Build history of the part. All positions in model axes, mm. Coordinates: 2 decimals unless noted, no trailing zeros. Order: outer loops, then holes, each group sorted by start corner. A loop starts at its lowest first (then second) coordinate and runs counter-clockwise, first axis right, second up. Notation, with made-up numbers: (35, 65.5) - (49, 65.5) arc R17 cw to (49, 74.5) - close; hole circle Ø8 at (43, 14.5). An arc over 180 degrees is marked (long way). One line per item, written item: value.
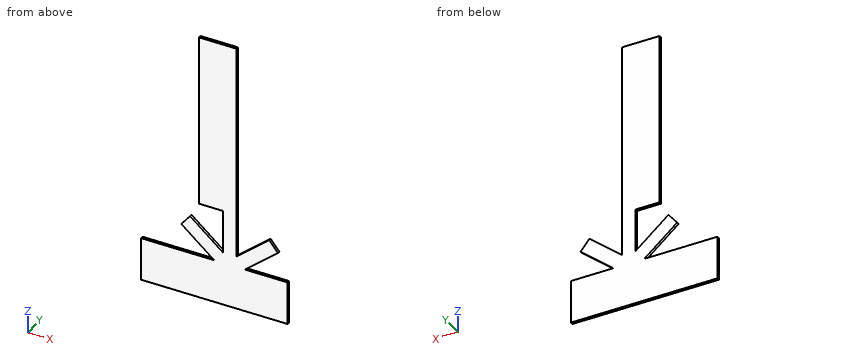
from build123d import *

# Parameters (mm, degrees)
F0_W     = 36.703
F0_H     = 50.8
F1_DEPTH = 3.175


with BuildPart() as f1:
    # F0 (on Front) → F1 (new body)
    with BuildSketch(Plane.XZ):
        Polygon((22.225, -101.6), (22.225, 101.6), (-22.225, 101.6), (-22.225, -101.6), (-6.35, -101.6), (6.35, -101.6), (6.35, -152.4), (-32.932004, -120.188757), (-43.346004, -132.888757), (-4.064, -165.1), (-54.864, -165.1), (-54.864, -215.9), (-4.064, -215.9), (14.2875, -215.9), (32.639, -215.9), (83.439, -215.9), (83.439, -165.1), (32.639, -165.1), (71.921004, -132.888757), (61.507004, -120.188757), (22.225, -152.4), align=None)
        with Locations((-73.2155, -190.5)):
            Rectangle(F0_W, F0_H)
    extrude(amount=F1_DEPTH)


solid = f1.part
1. Band-saw the part on A-A, the plane y = -2.1. Give the cut face in (x, z) (3 decimals).
Values found:
outline: (-91.567, -215.9) - (83.439, -215.9) - (83.439, -165.1) - (32.639, -165.1) - (71.921, -132.889) - (61.507, -120.189) - (22.225, -152.4) - (22.225, 101.6) - (-22.225, 101.6) - (-22.225, -101.6) - (6.35, -101.6) - (6.35, -152.4) - (-32.932, -120.189) - (-43.346, -132.889) - (-4.064, -165.1) - (-91.567, -165.1) - close
2. Band-saw the part on C-C, the plane z = 58.5. Give the cut face in (x, y) (3 decimals).
Values found:
outline: (-22.225, -3.175) - (22.225, -3.175) - (22.225, 0) - (-22.225, 0) - close
3. Flat gauge pin, fed straight in: P1, Ø1, axis at y = -2.5, z = 15, coming from the -X side (3 decimals). Where does the tip first touch, or does it go through?
Values found:
P1: stops at x = -22.225
4. Band-saw the part on B-B, the plane x = 1. Give the cut face in (y, z) (3 decimals).
Values found:
outline: (-3.175, -215.9) - (0, -215.9) - (0, -148.013) - (-3.175, -148.013) - close; (-3.175, -101.6) - (0, -101.6) - (0, 101.6) - (-3.175, 101.6) - close
5. Band-saw the part on D-D, the plane x = -78. Give the cut face in (y, z) (3 decimals), and give its area (3 significant figures).
Values found:
outline: (-3.175, -215.9) - (0, -215.9) - (0, -165.1) - (-3.175, -165.1) - close
area: 161 mm2
6. Probe line 1 along X through (y, z) = (-2.55, -123) (3 decimals); line 2 along Z through (x, y) = (-12, -0.8); line 3 along X through (y, z) = (-2.7, -39.5) (3 decimals). List the from-to ranges inside material, lowest first.
Values found:
line 1: x = -35.237 to -29.504, 6.35 to 22.225, 58.079 to 63.812
line 2: z = -215.9 to -165.1, -158.59 to -137.35, -101.6 to 101.6
line 3: x = -22.225 to 22.225
